Design review of the part built by this model. Coordinates are the model's own, in mm. A direction names the side the tool comes from. Round coordinates to 2 decimals unless told otherwise and drop trailing zeros. Loops run counter-clockwise (first coordinate to the right, second up) from the corner with the lowest first, then second, coordinate; pieces in that order, holes last. Notation, with made-up numbers: (23, 20.25) - (58, 20.25) arc R23 ccw to (58, 51.25) - close; hole circle Ø11 at (85, 11.5). An arc over 180 degrees is marked (long way). Use one line per item in the form item = value. Start each with the question number.
(1) For pin 1 (10 mm diameter, centred on y = -6.5, z = 17.5, fed in from +X); pin 2 (4 mm diameter, centred on x = -4, y = -10.5, fed in from +Z); pin 3 (3.5 mm diameter, centred on x = -2, z = -15, fed in from -Y), all flat-tipped, find the tip position at first contact; note any pin that passes through.
(2) Machinability: for faces 5 (the flat face through (-6.5, -2, -14.7)), 6 (the flat face through (6.5, -2, 18.5)), 7 (the flat face through (6.5, -2, -15.1)), 8 (the flat face through (-6.5, -2, 18.9)), which of the approach directions +Z, -Z, +X, -X, +Y, -Y give a long, thin tool a straight path to every point of the face, cutting with its end or side? Answer none if there is none.
(3) We need section A-A, the plane z = -9. Write out the cut boundary in (x, y).
(4) The part is to be moulded in two halves that separate along Y. For faces 1 (the conical face through (-0.7, -11.6, 19.5)), 2 (the flat face through (0, -3, 21)), 3 (the flat face through (-0.1, -0.5, 30)), 4 (the cylindrical face through (-1.626, -12.967, 2.612)), say which applies: released by +Y, released by -Y, zero draft, split by the parting line, or undercut.
(5) Wall thickness on probe 1 along Y at (x, z) = (5.5, 17); probe 2 along Y at (x, z) = (2.5, -12); probe 3 along Z at (x, y) = (-1.25, -8.75): over which ranges is each line inside the solid? List them lowest first. Write a range as [from, to].
from build123d import *

# Parameters (mm, degrees)
F0_W          = 15
F0_H          = 55
F1_DEPTH      = 3
F4_R          = 7.5
F5_DEPTH      = 20
F5_DEPTH_BACK = 5
F6_T1_DEPTH   = 25.2867319519
F6_T6_DEPTH   = 32.1433659759
F6_S7_R       = 7.5
F6_T8_DEPTH   = 18
F6_T14_DEPTH  = 32.1433659759
F6_S15_R      = 7.5
F6_T16_DEPTH  = 18
F6_T20_DEPTH  = 33.1433659759
F6_S21_R      = 7.5
F6_T22_DEPTH  = 18
F6_T26_DEPTH  = 33.1433659759
F6_S27_R      = 7.5
F6_T28_DEPTH  = 18
F7_DEPTH      = 25


# Not quite as in the source:
# - a fillet or chamfer that OpenCascade refuses, or shapes differently, is made with other operations: its cross-section is extruded or revolved along the edge and cut away or added


with BuildPart() as f1:
    # F0 (on Front) → F1 (new body)
    with BuildSketch(Plane.XZ):
        with Locations((0, 2.5)):
            Rectangle(F0_W, F0_H)
    extrude(amount=F1_DEPTH)

    # F4 (on face) → F5 (join, two sides)
    with BuildSketch(Plane(origin=(0, -1.5, 1.5), x_dir=(1, 0, 0), z_dir=(0, -0.7071067812, 0.7071067812))) as f5_sk:
        Circle(F4_R)
    extrude(amount=F5_DEPTH)
    extrude(f5_sk.sketch, amount=-F5_DEPTH_BACK)

    # F6: chamfer of 2 on 7 edges, made by hand

    # F6_s2 → F6_t1 (cut)
    with BuildSketch(Plane.YZ.offset(-12.6433659759)):
        Polygon((-1, 30), (-3, 28), (-3, 30), align=None)
        Polygon((-3, -23), (-1, -25), (-3, -25), align=None)
    extrude(amount=F6_T1_DEPTH, mode=Mode.SUBTRACT)


with BuildPart() as f6_tool4:
    # F6_s5 → F6_t6 (new body)
    with BuildSketch(Plane.XY.offset(35.1433659759)):
        Polygon((-5.5, -3), (-7.5, -1), (-7.5, -3), align=None)
    extrude(amount=-F6_T6_DEPTH)

    # F6_s7 → F6_t8 (cut, symmetric)
    with BuildSketch(Plane(origin=(0, -10.5358910397, 10.5358910397), x_dir=(1, 0, 0), z_dir=(0, 0.7071067812, -0.7071067812))):
        Circle(F6_S7_R)
    extrude(amount=F6_T8_DEPTH, both=True, mode=Mode.SUBTRACT)


with BuildPart() as f1_1:
    add(f1.part)

    # F6_t3: cut F6_tool4
    add(f6_tool4.part, mode=Mode.SUBTRACT)

    # F6_s9 → F6_t10 (revolve, cut)
    with BuildSketch(Plane(origin=(0, 0, 0), x_dir=(1, 0, 0), z_dir=(0, -0.7071067812, -0.7071067812))):
        Polygon((7.5, 20.1213203436), (5.5, 22.1213203436), (7.5, 22.1213203436), align=None)
    revolve(axis=Axis((0, -15.6421356237, 15.6421356237), (0, -0.7071067812, 0.7071067812)), mode=Mode.SUBTRACT)


with BuildPart() as f6_tool12:
    # F6_s13 → F6_t14 (new body)
    with BuildSketch(Plane.XY.offset(3)):
        Polygon((5.5, -3), (7.5, -1), (7.5, -3), align=None)
    extrude(amount=F6_T14_DEPTH)

    # F6_s15 → F6_t16 (cut, symmetric)
    with BuildSketch(Plane(origin=(0, -10.5358910397, 10.5358910397), x_dir=(1, 0, 0), z_dir=(0, 0.7071067812, -0.7071067812))):
        Circle(F6_S15_R)
    extrude(amount=F6_T16_DEPTH, both=True, mode=Mode.SUBTRACT)


with BuildPart() as f1_2:
    add(f1_1.part)

    # F6_t11: cut F6_tool12
    add(f6_tool12.part, mode=Mode.SUBTRACT)


with BuildPart() as f6_tool18:
    # F6_s19 → F6_t20 (new body)
    with BuildSketch(Plane.XY.offset(-30.1433659759)):
        Polygon((5.5, -3), (7.5, -1), (7.5, -3), align=None)
    extrude(amount=F6_T20_DEPTH)

    # F6_s21 → F6_t22 (cut, symmetric)
    with BuildSketch(Plane(origin=(0, 5.7982756057, -5.7982756057), x_dir=(1, 0, 0), z_dir=(0, 0.7071067812, -0.7071067812))):
        Circle(F6_S21_R)
    extrude(amount=F6_T22_DEPTH, both=True, mode=Mode.SUBTRACT)


with BuildPart() as f1_3:
    add(f1_2.part)

    # F6_t17: cut F6_tool18
    add(f6_tool18.part, mode=Mode.SUBTRACT)


with BuildPart() as f6_tool24:
    # F6_s25 → F6_t26 (new body)
    with BuildSketch(Plane.XY.offset(3)):
        Polygon((-5.5, -3), (-7.5, -1), (-7.5, -3), align=None)
    extrude(amount=-F6_T26_DEPTH)

    # F6_s27 → F6_t28 (cut, symmetric)
    with BuildSketch(Plane(origin=(0, 5.7982756057, -5.7982756057), x_dir=(1, 0, 0), z_dir=(0, 0.7071067812, -0.7071067812))):
        Circle(F6_S27_R)
    extrude(amount=F6_T28_DEPTH, both=True, mode=Mode.SUBTRACT)


with BuildPart() as f1_4:
    add(f1_3.part)

    # F6_t23: cut F6_tool24
    add(f6_tool24.part, mode=Mode.SUBTRACT)

    # F0 (on Front) → F7 (cut)
    with BuildSketch(Plane.XZ):
        with Locations((0, 2.5)):
            Rectangle(F0_W, F0_H)
    extrude(amount=-F7_DEPTH, mode=Mode.SUBTRACT)


solid = f1_4.part
Data:
q1.pin_1 = 7
q1.pin_2 = 19.31
q1.pin_3 = -3
q2.face_5 = -Z, -X, -Y
q2.face_6 = +Z, +X
q2.face_7 = -Z, +X, -Y
q2.face_8 = +Z, -X
q3.outline = (-7.5, -1) - (-5.5, -3) - (5.5, -3) - (7.5, -1) - (7.5, 0) - (-7.5, 0) - close
q4.face_1 = released by -Y
q4.face_2 = undercut
q4.face_3 = zero draft
q4.face_4 = undercut
q5.probe_1 = [-13.56, -9.79], [-3, 0]
q5.probe_2 = [-3, 0]
q5.probe_3 = [-1.71, 19.21]
